from build123d import *

# Parameters (mm, degrees)
SWEEP1_PROFILE_R = 25
SWEEP4_PROFILE_R = 25
LPATTERN1_COUNT  = 7
LPATTERN1_PITCH  = 205


with BuildPart() as part:
    # Sweep1: sweep along a curve in space
    with BuildLine() as sweep1_path:
        Line((698, 673.348237879, 1724.841016462), (548, 2173.348237879, 1352.615298417))
        Line((548, 2173.348237879, 1352.615298417), (548, 2173.348237879, 129.165241299))
        Line((548, 2173.348237879, 129.165241299), (747.126637555, 679.898456219, -274.544806265))
    # Sweep1 profile (on start of the path) → Sweep1 (sweep)
    with BuildSketch(Plane(origin=(698, 673.348237879, 1724.841016462), x_dir=(0, 0.24084577238006388, 0.9705634002612351), z_dir=(-0.09660241237961904, 0.9660241237961907, -0.23971934875232764))):
        Circle(SWEEP1_PROFILE_R)
    sweep(path=sweep1_path.line, transition=Transition.RIGHT)


with BuildPart() as body_2:
    # Mirror2: mirrored copy
    add(part.part.mirror(Plane(origin=(0, 0, 0), x_dir=(0, 0, 1), z_dir=(1, 0, 0))))


with BuildPart() as part_1:
    add(part.part)

    add(body_2.part)  # Sweep4 merges body 2
    # Sweep4: sweep along a curve in space
    with BuildLine() as sweep4_path:
        Line((523.124060053, 2170.860746823, 1352.61537863), (-523.124060053, 2170.860746823, 1352.61537863))
    # Sweep4 profile (on start of the path) → Sweep4 (sweep)
    with BuildSketch(Plane(origin=(523.124060053, 2170.860746823, 1352.61537863), x_dir=(0, -1, 0), z_dir=(-1, 0, 0))):
        Circle(SWEEP4_PROFILE_R)
    sweep4 = sweep(path=sweep4_path.line)

    # LPattern1: Sweep4 ×7
    with Locations(*[(0, 0, -i * LPATTERN1_PITCH) for i in range(1, LPATTERN1_COUNT)]):
        add(sweep4)


solid = part_1.part
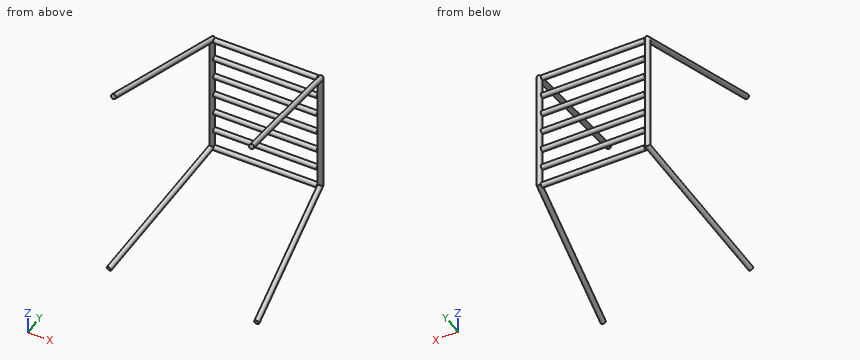
Read the model definition and answer for the solid it produces. Units are mm, in the model's axes. Give positions to 0.01 mm unless a question says otherwise; leave off trailing zeros. Write each loop counter-clockwise with the first axis right and the second up, starting at its lowest first coordinate (ties: lowest second). Pieces come first, ordered by that corner, then holes. Notation, with made-up numbers: M 0,38.5 L 23,38.5 A26 cw 23,54.5 Z; hole C 21,-22.5 d4. An arc over 180 degrees is marked long. One line per item, written item: value. Start each with the question number.
(1) Find the intervals of material crossed by line 1 (X direction, y = 1130, z = -160.5); line 2 (Z direction, x = -596.5, y = 1813); line 3 (Y direction, x = 327, z = 718.5), in increasing order.
(2) Find section B-B (z = 181). Determine the outline of the cut face in (x, y).
(3) Flat-ended cylindrical pins translate along their axes: pin 1 Ø10 at (y, z) = (2183.5, 1146) entering from +X; pin 2 Ø16 at (y, z) = (2184, 1149.5) entering from -X; pin 3 Ø20 at (y, z) = (2157.5, 1136) entering from -X. Find the tip coordinate at first contact, or state that the pin passes through.
(4) Find section C-C (y = 1136). Give the number of separate pieces and of enclosed holes in the cut face, plus the area to 3 significant figures.
(5) Find section A-A (x = -377). Determine the outline of the cut face in (y, z).
Results below:
1. line 1: x = -711.46 to -663.28, 663.28 to 711.46
1. line 2: z = 5.86 to 57.62, 1419.98 to 1464.7
1. line 3: y = 2154.75 to 2186.97
2. outline: C -548,2173.35 d50; C 548,2173.35 d50
3. pin 1: stops at x = 572.46
3. pin 2: stops at x = -572.86
3. pin 3: stops at x = -572.31
4. separate pieces: 4
4. enclosed holes: 0
4. area: 8,170 mm^2
5. outline: C 2170.86,122.62 d50; C 2170.86,327.62 d50; C 2170.86,532.62 d50; C 2170.86,737.62 d50; C 2170.86,942.62 d50; C 2170.86,1147.62 d50; C 2170.86,1352.62 d50
